CAD build for the part. Positions are in the model's coordinates, mm. Coordinates: 2 decimals unless noted, no trailing zeros. Loops run counter-clockwise (first coordinate to the right, second up) from the corner with the lowest first, then second, coordinate; pieces in that order, holes last. Notation, with made-up numbers: (84, -39) -> (91, -39) arc R15 cw to (91, -14) -> close; hole circle Ø6 at (-31.5, 77). An arc over 180 degrees is marked (long way). Write each question's results on one line, items separated by ' | '.
from build123d import *

# Parameters (mm, degrees)
SKETCH_1_W          = 10
SKETCH_1_H          = 10
SKETCH_1_W_2        = 8
SKETCH_1_H_2        = 8
EXTRUDE_1_DEPTH     = 225
SKETCH_2_R          = 2
CUT_EXTRUDE_1_DEPTH = 226.277606521
SKETCH_3_R          = 2
CUT_EXTRUDE_2_DEPTH = 226.277606521


with BuildPart() as part:
    # ｽｹｯﾁ1 → 押し出し-薄板1 (new body)
    with BuildSketch(Plane(origin=(0, 0, 0), x_dir=(0, 0, -1), z_dir=(1, 0, 0))):
        Rectangle(SKETCH_1_W, SKETCH_1_H)
        Rectangle(SKETCH_1_W_2, SKETCH_1_H_2, mode=Mode.SUBTRACT)
    extrude(amount=EXTRUDE_1_DEPTH)

    # ｽｹｯﾁ2 → ｶｯﾄ - 押し出し1 (cut, through all)
    with BuildSketch(Plane.XY.offset(5)):
        with Locations((37.5, 0)):
            Circle(SKETCH_2_R)
        with Locations(Location((187.5, 0, 0), (0, 0, 90))):
            Circle(SKETCH_2_R)
        with Locations((112.5, 0)):
            Circle(SKETCH_2_R)
        with Locations((12.5, 0)):
            Circle(SKETCH_2_R)
        with Locations(Location((212.5, 0, 0), (0, 0, 90))):
            Circle(SKETCH_2_R)
    extrude(amount=-CUT_EXTRUDE_1_DEPTH, mode=Mode.SUBTRACT)

    # ｽｹｯﾁ3 → ｶｯﾄ - 押し出し2 (cut, through all)
    with BuildSketch(Plane(origin=(0, 5, 0), x_dir=(1, 0, 0), z_dir=(0, 1, 0))):
        with Locations(Location((5, 0, 0), (0, 0, 270))):
            Circle(SKETCH_3_R)
        with Locations(Location((220, 0, 0), (0, 0, 270))):
            Circle(SKETCH_3_R)
        with Locations(Location((100, 0, 0), (0, 0, 270))):
            Circle(SKETCH_3_R)
        with Locations(Location((125, 0, 0), (0, 0, 270))):
            Circle(SKETCH_3_R)
    extrude(amount=-CUT_EXTRUDE_2_DEPTH, mode=Mode.SUBTRACT)


solid = part.part
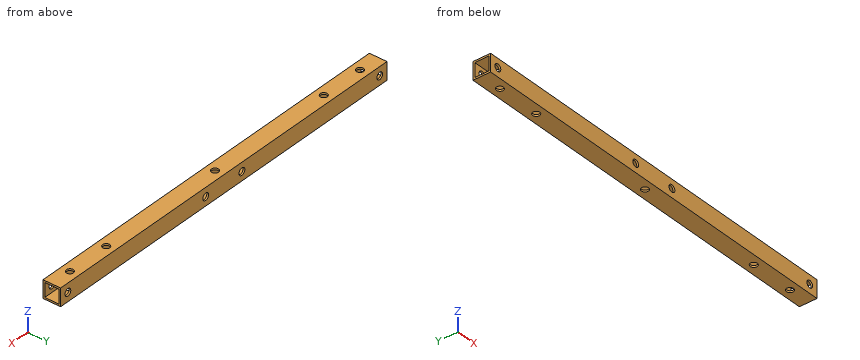
1) Slice it at A-A (x = 212.5). Write the cut outline in (y, z), then the cut area to 3 significant figures.
Outcome:
outline: (-5, -5) -> (-2, -5) -> (-2, -4) -> (-4, -4) -> (-4, 4) -> (-2, 4) -> (-2, 5) -> (-5, 5) -> close; (2, -5) -> (5, -5) -> (5, 5) -> (2, 5) -> (2, 4) -> (4, 4) -> (4, -4) -> (2, -4) -> close | area: 28.0 mm^2
2) Drill centre lines: L1, parallel to X at y = -4.7, z = 0; L2, parallel to Y at x = 48, z = -1.25. Where is each one in solid material? Low to high. Write a range as from..to.
Outcome:
L1: x = 0..3, 7..98, 102..123, 127..218, 222..225 | L2: y = -5..-4, 4..5
3) Slice it at B-B (y = 0). Count the separate pieces of the cut face and the enclosed holes in it, then the cut area to 3 significant figures.
Outcome:
separate pieces: 12 | enclosed holes: 0 | area: 410 mm^2
4) Slice it at C-C (x = 55). Write the cut outline in (y, z).
Outcome:
outline: (-5, -5) -> (5, -5) -> (5, 5) -> (-5, 5) -> close; hole (-4, -4) -> (4, -4) -> (4, 4) -> (-4, 4) -> close
